Can you work these out from the model? Positions are in its coordinate system, mm. Give positions to 0.01 mm unless a question says otherwise; leave off trailing zeros. Write each loop counter-clockwise with the first axis right and the second up, starting at its lowest first coordinate (ties: lowest second). Pieces come first, ordered by that corner, then holes.
from build123d import *

# Parameters (mm, degrees)
F0_W     = 2082.8
F0_H     = 161.925
F1_DEPTH = 44.45
F2_W     = 1981.2
F2_H     = 9.525
F3_DEPTH = 12.7
F4_W     = 1981.2
F4_H     = 9.525
F5_DEPTH = 12.7
F6_W     = 2082.8
F6_H     = 19.05
F7_DEPTH = 12.7
F8_W     = 12.7
F8_H     = 25.4
F9_DEPTH = 31.751


with BuildPart() as f1:
    # F0 (on Top) → F1 (new body)
    with BuildSketch(Plane.XY):
        with Locations((80.949743, -511.85186)):
            Rectangle(F0_W, F0_H)
    extrude(amount=F1_DEPTH)

    # F2 (on face) → F3 (cut)
    with BuildSketch(Plane(origin=(0, 0, 0), x_dir=(1, 0, 0), z_dir=(0, 0, -1))):
        Polygon((-960.450257, 592.81436), (-960.450257, 430.88936), (-909.650257, 430.88936), (-909.650257, 583.28936), (-909.650257, 592.81436), align=None)
        with Locations((80.949743, 588.05186)):
            Rectangle(F2_W, F2_H)
        Polygon((1071.549743, 592.81436), (1071.549743, 583.28936), (1071.549743, 430.88936), (1122.349743, 430.88936), (1122.349743, 592.81436), align=None)
    extrude(amount=-F3_DEPTH, mode=Mode.SUBTRACT)

    # F4 (on face) → F5 (cut)
    with BuildSketch(Plane.XY.offset(44.45)):
        Polygon((1122.349743, -430.88936), (1071.549743, -430.88936), (1071.549743, -583.28936), (1071.549743, -592.81436), (1122.349743, -592.81436), align=None)
        with Locations((80.949743, -588.05186)):
            Rectangle(F4_W, F4_H)
        Polygon((-909.650257, -592.81436), (-909.650257, -583.28936), (-909.650257, -430.88936), (-960.450257, -430.88936), (-960.450257, -592.81436), align=None)
    extrude(amount=-F5_DEPTH, mode=Mode.SUBTRACT)

    # F6 (on face) → F7 (cut)
    with BuildSketch(Plane(origin=(0, -430.88936, 0), x_dir=(-1, 0, 0), z_dir=(0, 1, 0))):
        with Locations((-80.949743, 22.225)):
            Rectangle(F6_W, F6_H)
    extrude(amount=-F7_DEPTH, mode=Mode.SUBTRACT)

    # F8 (on face) → F9 (cut, through all)
    with BuildSketch(Plane(origin=(0, 0, 12.7), x_dir=(1, 0, 0), z_dir=(0, 0, -1))):
        with Locations((-935.050257, 516.61436)):
            Rectangle(F8_W, F8_H)
        with Locations((1096.949743, 516.61436)):
            Rectangle(F8_W, F8_H)
    extrude(amount=-F9_DEPTH, mode=Mode.SUBTRACT)


solid = f1.part
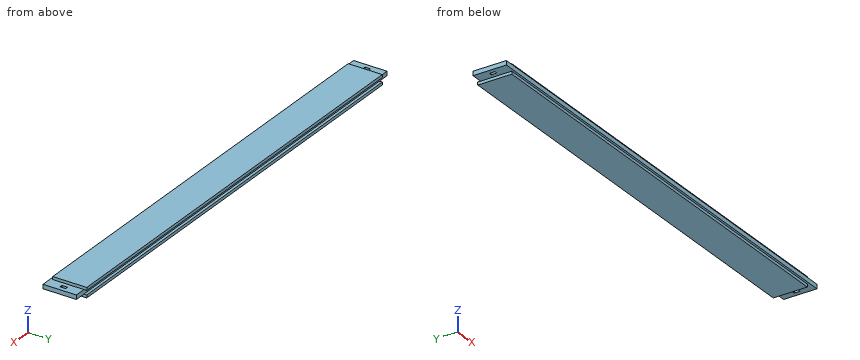
(1) Imagine slicing it at A-A, the plane z = 25. Write out the boundary of the cut face in (x, y), plus the area to 3 significant figures.
Returned:
outline: (-960.45, -592.81) - (1122.35, -592.81) - (1122.35, -443.59) - (-960.45, -443.59) - close; hole (-941.4, -529.31) - (-928.7, -529.31) - (-928.7, -503.91) - (-941.4, -503.91) - close; hole (1090.6, -529.31) - (1103.3, -529.31) - (1103.3, -503.91) - (1090.6, -503.91) - close
area: 310,000 mm2
(2) Imagine slicing it at B-B, the plane y = -559.5. Write out the boundary of the cut face in (x, z), plus the area to 3 significant figures.
Returned:
outline: (-960.45, 12.7) - (-909.65, 12.7) - (-909.65, 0) - (1071.55, 0) - (1071.55, 12.7) - (1122.35, 12.7) - (1122.35, 31.75) - (1071.55, 31.75) - (1071.55, 44.45) - (-909.65, 44.45) - (-909.65, 31.75) - (-960.45, 31.75) - close
area: 90,000 mm2
(3) Will these pins go through, and if not, where does the flat tip stop? P1, Ø6.5, axis at x = -234, z = 7, coming from the -Y side; P2, Ø10, axis at y = -485, z = 4, coming from the +X side; P3, Ø10, axis at y = -507, z = 4, coming from the -X side.
Returned:
P1: stops at y = -583.29
P2: stops at x = 1071.55
P3: stops at x = -909.65
(4) Imagine slicing it at C-C, the plane x = 493.5. Write out the boundary of the cut face in (y, z).
Returned:
outline: (-592.81, 12.7) - (-583.29, 12.7) - (-583.29, 0) - (-430.89, 0) - (-430.89, 12.7) - (-443.59, 12.7) - (-443.59, 31.75) - (-430.89, 31.75) - (-430.89, 44.45) - (-583.29, 44.45) - (-583.29, 31.75) - (-592.81, 31.75) - close
(5) If I drill on L1, parallel to Z at x = 665, y = -439.5; L2, parallel to Y at x = -691.5, z = 41; L3, parallel to Y at x = -863, z = 25.5, over which ranges is the centre line in solid material (lowest first)?
Returned:
L1: z = 0 to 12.7, 31.75 to 44.45
L2: y = -583.29 to -430.89
L3: y = -592.81 to -443.59
